Design review of the part built by this model. Coordinates are the model's own, in mm. A direction names the side the tool comes from. Coordinates: 2 decimals unless noted, no trailing zeros. Loops run counter-clockwise (first coordinate to the right, second up) from the corner with the lowest first, then second, coordinate; pieces in that order, holes last. Notation, with made-up numbers: M 9.5,2.5 L 57.5,2.5 A23 cw 57.5,15.5 Z; hole C -9.75,86.25 d6. An arc over 180 degrees is marked long. Answer as a JSON object with one key per item and string values. Group by question number.
1. Consider section D-D (y = 0). Count the separate pieces of the cut face and the enclosed holes in it, then the cut area to 3 significant figures.
2. Consider section B-B (z = -96.5). State the section outline as (x, y) points, then the cut area to 3 significant figures.
3. Consider section C-C (z = 260). State the section outline as (x, y) points, then the cut area to 3 significant figures.
4. Draft analysis for pull direction Y (two halves, no side actions). For faces 1 (the flat face through (186, 240, 2)), 2 (the flat face through (137.351, 130.345, 1.988)), 3 (the cylindrical face through (-4.336, -19.524, -120.42)), 4 (the cylindrical face through (39.53, 92.4, 245.29)), state which applies: +Y half, -Y half, draft (parallel to the pull), parting line (faces both ways), or undercut.
5. Insertion check: pin 1 (4.5 mm diameter, centred on y = 48, z = 178.5, fed in from +X); pin 2 (18 mm diameter, centred on x = 0, z = 260, fed in from -Y); pin 3 (10 mm diameter, centred on y = 123, z = 110.5, fed in from -X); pin 4 (8 mm diameter, centred on x = 127, y = 126, fed in from -Z). Each pin has a flat end and moves straight along its axis. Give the tip position at first contact, or say it passes through.
6. To check wall thickness, follow probe 1 along Y at (x, z) = (44.5, 201.5); probe 2 along Z at (x, y) = (14.5, 24); probe 3 along Y at (x, z) = (0, -107). State the ranges of each line that lie inside material, in increasing order.
7. Consider section A-A (z = 169). State the section outline as (x, y) points, then the cut area to 3 significant figures.
8. Machinability: for faces 5 (the flat face through (1, 40, 205)), 6 (the flat face through (-55, 47, 170)), 7 (the flat face through (55, 47, 170)), which of the approach directions +Z, -Z, +X, -X, +Y, -Y give a long, thin tool a straight path to every point of the face, cutting with its end or side? Answer none if there is none.
from build123d import *

# Parameters (mm, degrees)
SKETCH1_R             = 20
BOSS_EXTRUDE1_DEPTH   = 150
BOSS_EXTRUDE2_START   = 40
SKETCH2_R             = 15
BOSS_EXTRUDE2_DEPTH   = 60
SKETCH3_W             = 178.732333714
SKETCH3_H             = 30
CUT_EXTRUDE1_DEPTH    = 150
SKETCH4_W             = 180
SKETCH4_H             = 180.454063709
CUT_EXTRUDE2_DEPTH    = 170
CHAMFER1_SIZE         = 4
CHAMFER1_SIZE2        = 21.339042193
CHAMFER1_EDGE_2_SIZE  = 4
CHAMFER1_EDGE_2_SIZE2 = 21.339042193
FILLET1_R             = 4
FILLET2_R             = 8


with BuildPart() as part:
    # Sketch1 → Boss-Extrude1 (new, symmetric)
    with BuildSketch(Plane.XY):
        with BuildLine():
            Line((175.499287748, 240), (195.959179423, 240))
            ThreePointArc((195.959179423, 240), (182.049998135, 197.188176092), (158.918539009, 158.571428571))
            Line((158.918539009, 158.571428571), (23.837780851, -18.214285714))
            ThreePointArc((23.837780851, -18.214285714), (0, -30), (-23.837780851, -18.214285714))
            Line((-23.837780851, -18.214285714), (-158.918539009, 158.571428571))
            ThreePointArc((-158.918539009, 158.571428571), (-182.049998135, 197.188176092), (-195.959179423, 240))
            Line((-195.959179423, 240), (-175.499287748, 240))
            ThreePointArc((-175.499287748, 240), (0, 100), (175.499287748, 240))
        make_face()
        Circle(SKETCH1_R, mode=Mode.SUBTRACT)
    extrude(amount=BOSS_EXTRUDE1_DEPTH, both=True)

    # Sketch2 → Boss-Extrude2 (add)
    with BuildSketch(Plane(origin=(0, 0, 0), x_dir=(1, 0, 0), z_dir=(0, 1, 0)).offset(BOSS_EXTRUDE2_START)):
        with BuildLine():
            Line((0, -150), (55, -150))
            Line((55, -150), (55, -190))
            Line((55, -190), (45.381291361, -223.665480236))
            ThreePointArc((45.381291361, -223.665480236), (39.450512778, -245.597555378), (34.14492902, -267.689201664))
            ThreePointArc((34.14492902, -267.689201664), (0, -295), (-34.14492902, -267.689201664))
            ThreePointArc((-34.14492902, -267.689201664), (-39.450512778, -245.597555378), (-45.381291361, -223.665480236))
            Line((-45.381291361, -223.665480236), (-55, -190))
            Line((-55, -190), (-55, -150))
            Line((-55, -150), (0, -150))
        make_face()
        with Locations(Location((0, -260, 0), (0, 0, 270))):
            Circle(SKETCH2_R, mode=Mode.SUBTRACT)
    extrude(amount=BOSS_EXTRUDE2_DEPTH)

    # Sketch3 → Cut-Extrude1 (cut)
    with BuildSketch(Plane(origin=(55, 0, 0), x_dir=(0, 0, -1), z_dir=(1, 0, 0))):
        with Locations((-239.366166857, 70)):
            Rectangle(SKETCH3_W, SKETCH3_H)
    extrude(amount=-CUT_EXTRUDE1_DEPTH, mode=Mode.SUBTRACT)

    # Sketch4 → Cut-Extrude2 (cut, symmetric)
    with BuildSketch(Plane(origin=(0, 0, 0), x_dir=(0, 0, -1), z_dir=(1, 0, 0))):
        with Locations((0, 4.772968145)):
            Rectangle(SKETCH4_W, SKETCH4_H)
    extrude(amount=CUT_EXTRUDE2_DEPTH, both=True, mode=Mode.SUBTRACT)

    # Chamfer1
    chamfer1_edges = [part.edges().sort_by_distance(p)[0] for p in [
        (-110.344044156, 95, 0),
    ]]
    chamfer1_side = [part.faces().sort_by_distance(p)[0] for p in [
        (0, 95, 0),
    ]]
    chamfer(chamfer1_edges, length=CHAMFER1_SIZE, length2=CHAMFER1_SIZE2, reference=chamfer1_side[0])

    # Chamfer1 edge 2
    chamfer1_edge_2_edges = [part.edges().sort_by_distance(p)[0] for p in [
        (110.344044156, 95, 0),
    ]]
    chamfer1_edge_2_side = [part.faces().sort_by_distance(p)[0] for p in [
        (0, 95, 0),
    ]]
    chamfer(chamfer1_edge_2_edges, length=CHAMFER1_EDGE_2_SIZE, length2=CHAMFER1_EDGE_2_SIZE2, reference=chamfer1_edge_2_side[0])

    # Fillet1
    fillet1_edges = [part.edges().sort_by_distance(p)[0] for p in [
        (0, 95, 90),
        (0, 95, -90),
    ]]
    fillet(fillet1_edges, radius=FILLET1_R)

    # Fillet2
    fillet2_edges = [part.edges().sort_by_distance(p)[0] for p in [
        (182.049998135, 197.188176092, -150),
        (91.37815993, 70.178571429, -150),
        (0, -30, -150),
        (182.049998135, 197.188176092, 150),
        (-182.049998135, 197.188176092, 150),
        (-91.37815993, 70.178571429, 150),
        (0, -30, 150),
        (-91.37815993, 70.178571429, -150),
        (91.37815993, 70.178571429, 150),
        (-182.049998135, 197.188176092, -150),
    ]]
    fillet(fillet2_edges, radius=FILLET2_R)


solid = part.part
Findings below:
{
 "1": {"separate pieces": "4", "enclosed holes": "0", "area": "4,190 mm^2"},
 "2": {"outline": "M -195.96,240 A200 ccw -158.92,158.57 L -23.84,-18.21 A30 ccw 23.84,-18.21 L 158.92,158.57 A200 ccw 195.96,240 L 175.5,240 A180 cw -175.5,240 Z; hole C 0,0 d40", "area": "24,300 mm^2"},
 "3": {"outline": "M -35.92,40 L -15,40 L -15,55 L -35.92,55 Z; M -35.92,85 L -15,85 L -15,100 L -35.92,100 Z; M 15,40 L 35.92,40 L 35.92,55 L 15,55 Z; M 15,85 L 35.92,85 L 35.92,100 L 15,100 Z", "area": "1,250 mm^2"},
 "4": {"face 1": "+Y half", "face 2": "-Y half", "face 3": "undercut", "face 4": "draft"},
 "5": {"pin 1": "stops at x = 55", "pin 2": "passes through", "pin 3": "stops at x = -135.56", "pin 4": "stops at z = -150"},
 "6": {"probe 1": "y = 40 to 55, 85 to 100", "probe 2": "z = -150 to -90, 90 to 150", "probe 3": "y = -30 to -20, 20 to 100"},
 "7": {"outline": "M -55,40 L 55,40 L 55,55 L -55,55 Z; M -55,85 L 55,85 L 55,100 L -55,100 Z", "area": "3,300 mm^2"},
 "8": {"face 5": "+Z, +X, -X, -Y", "face 6": "+Z, -X, +Y, -Y", "face 7": "+Z, +X, +Y, -Y"}
}
